Source: CAD feature listing. Evaluate the final solid. Frame: model axes, mm. Face numbers are marked on the shaded views. Round coordinates to 2 decimals unless told otherwise and drop trailing zeros. Order: outer loops, then holes, each group sorted by start corner. A loop starts at its lowest first (then second) coordinate and runs counter-clockwise, first axis right, second up. Notation, with made-up numbers: (72.25, 63.5) - (93.25, 63.5) arc R23 cw to (93.25, 74.5) - close; hole circle Ø1 at (21, 0.5). An arc over 180 degrees is marked (long way). Return JSON: item names as keys, results as strings. Group by question number.
1) Section C-C, the plane z = 4. Return loops of the section in (x, y) (1 decimal).
2) Section B-B, the plane z = 2.9. Give the number of separate pieces and of enclosed holes in the cut face, plus the area to 3 significant figures.
3) Mould query, pull axis Y, two halves, no side actions, for the marked faces 1, 2 and 3. Classes: pulls with the +Y half, pulls with the -Y half, needs draft (parallel to the pull), parting line crosses it, or undercut.
4) Section A-A, the plane y = 0. Return loops of the section in (x, z).
5) Ray query, line 1 (Y direction, x = 0, z = 3.45); line 2 (Y direction, x = 0, z = 4); line 3 (Z direction, x = -11, y = 2.75). Return the intervals inside material, ascending. Write a range as from..to.
```python
from build123d import *

# Parameters (mm, degrees)
BOSS_EXTRUDE1_DEPTH        = 4.7625
CUT_EXTRUDE1_DEPTH         = 1.3335
F_1_8_0_1250_DOWEL_HOLE1_D = 3.175
FILLET1_R                  = 1.27


with BuildPart() as part:
    # Sketch1 → Boss-Extrude1 (new body)
    with BuildSketch(Plane.XY):
        with BuildLine():
            Line((-9.921875, 3.99643469), (-1.5875, 6.148361062))
            ThreePointArc((-1.5875, 6.148361062), (6.35, 0), (-1.5875, -6.148361062))
            Line((-1.5875, -6.148361062), (-9.921875, -3.99643469))
            ThreePointArc((-9.921875, -3.99643469), (-13.0175, 0), (-9.921875, 3.99643469))
        make_face()
    extrude(amount=BOSS_EXTRUDE1_DEPTH)

    # Sketch2 → Cut-Extrude1 (cut)
    with BuildSketch(Plane(origin=(0, 0, 0), x_dir=(-1, 0, 0), z_dir=(0, 0, -1))):
        with BuildLine():
            Line((9.921875, 3.99643469), (1.5875, 6.148361062))
            ThreePointArc((1.5875, 6.148361062), (-6.35, 0), (1.5875, -6.148361062))
            Line((1.5875, -6.148361062), (9.921875, -3.99643469))
            ThreePointArc((9.921875, -3.99643469), (13.0175, 0), (9.921875, 3.99643469))
        make_face()
    extrude(amount=-CUT_EXTRUDE1_DEPTH, mode=Mode.SUBTRACT)

    # 1/8 (0.1250) Dowel Hole1 (through all)
    with Locations(Plane(origin=(0, 0, 1.3335), x_dir=(-1, 0, 0), z_dir=(0, 0, -1))):
        with Locations((8.89, 0), (0, 0)):
            Hole(F_1_8_0_1250_DOWEL_HOLE1_D / 2)

    # Fillet1
    fillet1_edges = [part.edges().sort_by_distance(p)[0] for p in [
        (6.35, 0, 4.7625),
        (-5.7546875, 5.072397876, 4.7625),
        (-13.0175, 0, 4.7625),
        (-5.7546875, -5.072397876, 4.7625),
    ]]
    fillet(fillet1_edges, radius=FILLET1_R)


solid = part.part
```
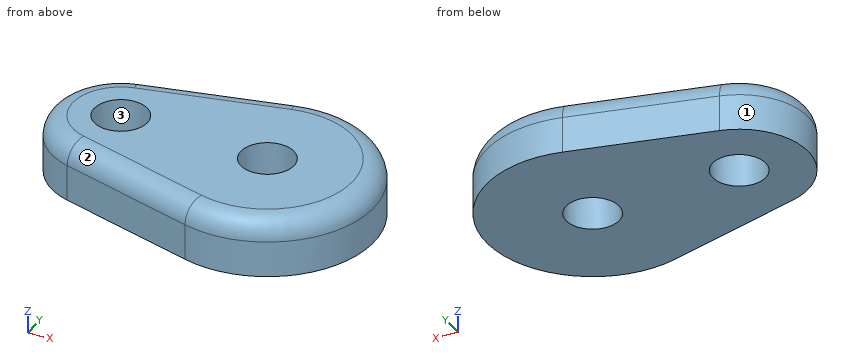
Geometry check:
{
 "1": {"outline": "(-9.9, -3.9) - (-1.6, -6) arc R6.2 ccw (long way) to (-1.6, 6) - (-9.9, 3.9) arc R4 ccw to start; hole circle Ø3.2 at (-8.9, 0); hole circle Ø3.2 at (0, 0)"},
 "2": {"separate pieces": "1", "enclosed holes": "2", "area": "170 mm2"},
 "3": {"face 1": "parting line crosses it", "face 2": "pulls with the -Y half", "face 3": "undercut"},
 "4": {"outline": "(-13.02, 1.33) - (-10.48, 1.33) - (-10.48, 4.76) - (-11.75, 4.76) arc R1.27 ccw to (-13.02, 3.49) - close; (-7.3, 1.33) - (-1.59, 1.33) - (-1.59, 4.76) - (-7.3, 4.76) - close; (1.59, 1.33) - (6.35, 1.33) - (6.35, 3.49) arc R1.27 ccw to (5.08, 4.76) - (1.59, 4.76) - close"},
 "5": {"line 1": "-6.35..-1.59, 1.59..6.35", "line 2": "-6.24..-1.59, 1.59..6.24", "line 3": "1.33..4.61"}
}
